Part model, mm, in its own coordinate system. Face numbers are marked on the shaded views. A direction names the side the tool comes from. Round coordinates to 2 decimals unless told otherwise and drop trailing zeros. Loops run counter-clockwise (first coordinate to the right, second up) from the corner with the lowest first, then second, coordinate; pieces in that order, holes last. Notation, with made-up numbers: M -25,-4 L 17,-4 A28 cw 17,22 Z; hole C 38,-17.75 d7. An arc over 180 degrees is marked long. Put each result on its own line as item: value. Start each with the question number.
```python
from build123d import *

# Parameters (mm, degrees)
SKETCH_1_W                  = 86
SKETCH_1_H                  = 43
EXTRUDE_1_DEPTH             = 39.5
EXTRUDE_2_DEPTH             = 5
SKETCH_3_W                  = 80.6
SKETCH_3_H                  = 40.2
CUT_EXTRUDE_1_DEPTH         = 43.6
HOLE_WIZARD_8_3_8_3_1_D     = 8.3
HOLE_WIZARD_8_3_8_3_1_DEPTH = 3.2
FILLET_1_R                  = 3
EXTRUDE_START               = -4
SKETCH_6_R                  = 4.15
EXTRUDE_3_DEPTH             = 4
SKETCH_10_W                 = 2.2
SKETCH_10_H                 = 43
EXTRUDE_5_DEPTH             = 42
FILLET_2_R                  = 2


with BuildPart() as part:
    # Эскиз1 → Бобышка-Вытянуть1 (new body)
    with BuildSketch(Plane.XY.offset(22.25)):
        with Locations((47, 0)):
            Rectangle(SKETCH_1_W, SKETCH_1_H)
    extrude(amount=-EXTRUDE_1_DEPTH)

    # Эскиз2 → Бобышка-Вытянуть2 (add)
    with BuildSketch(Plane(origin=(0, 0, -17.25), x_dir=(-1, 0, 0), z_dir=(0, 0, -1))):
        with BuildLine():
            Line((-90, -21.5), (-90, -16.5))
            ThreePointArc((-90, -16.5), (-104, 0), (-90, 16.5))
            Line((-90, 16.5), (-90, 21.5))
            Line((-90, 21.5), (-4, 21.5))
            Line((-4, 21.5), (-4, -21.5))
            Line((-4, -21.5), (-90, -21.5))
        make_face()
        with BuildLine():
            Line((-90, -12.428366172), (-90, 12.428366172))
            ThreePointArc((-90, 12.428366172), (-100, 0), (-90, -12.428366172))
        make_face(mode=Mode.SUBTRACT)
    extrude(amount=EXTRUDE_2_DEPTH)

    # Эскиз3 → Вырез-Вытянуть1 (cut)
    with BuildSketch(Plane.XY.offset(22.25)):
        with Locations((48.3, 0)):
            Rectangle(SKETCH_3_W, SKETCH_3_H)
    extrude(amount=-CUT_EXTRUDE_1_DEPTH, mode=Mode.SUBTRACT)

    # Диаметр отверстия Ø8.3 (8.3)1
    with Locations(Plane.ZY.offset(-4)):
        with Locations((0, 0)):
            Hole(HOLE_WIZARD_8_3_8_3_1_D / 2, depth=HOLE_WIZARD_8_3_8_3_1_DEPTH)

    # Скругление1
    fillet_1_edges = [part.edges().sort_by_distance(p)[0] for p in [
        (4, -21.5, 0),
        (4, 21.5, 0),
    ]]
    fillet(fillet_1_edges, radius=FILLET_1_R)

    # Эскиз6 → Бобышка-Вытянуть3 (add)
    with BuildSketch(Plane.ZY.offset(-4).offset(EXTRUDE_START)):
        Circle(SKETCH_6_R)
    extrude(amount=EXTRUDE_3_DEPTH)

    # Эскиз10 → Бобышка-Вытянуть5 (add)
    with BuildSketch(Plane(origin=(0, 0, -22.25), x_dir=(-1, 0, 0), z_dir=(0, 0, -1))):
        with Locations((-47.4, 0)):
            Rectangle(SKETCH_10_W, SKETCH_10_H)
    extrude(amount=-EXTRUDE_5_DEPTH)

    # Скругление2
    fillet_2_edges = [part.edges().sort_by_distance(p)[0] for p in [
        (27.15, -20.1, -21.35),
        (88.6, -20.1, 0.45),
        (8, 0, -21.35),
        (8, -20.1, 0.45),
        (68.55, 20.1, -21.35),
        (8, 20.1, 0.45),
        (88.6, 0, -21.35),
        (68.55, -20.1, -21.35),
        (27.15, 20.1, -21.35),
        (48.5, 0, -21.35),
        (46.3, 0, -21.35),
        (90, 21.5, 0),
        (46.3, -20.1, -0.8),
        (46.3, 20.1, -0.8),
        (48.5, -20.1, -0.8),
        (48.5, 20.1, -0.8),
    ]]
    fillet(fillet_2_edges, radius=FILLET_2_R)


solid = part.part
```
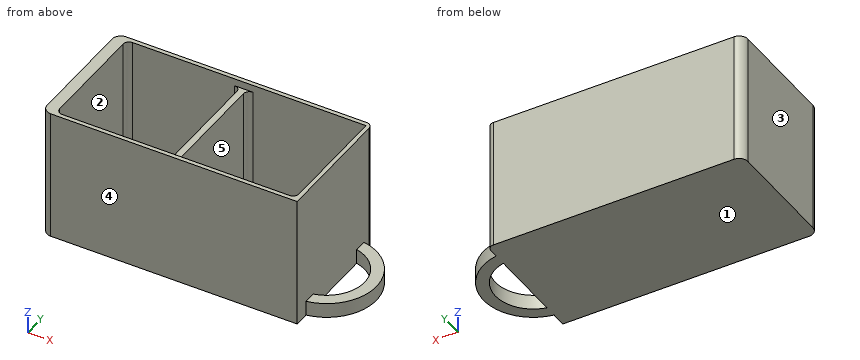
1. Cut at B-B, the plane y = 7. Give the cut face in (x, z).
2. Mould opens along X. For the marked faces 3, 4 and 5 say: released by +X, released by -X, zero draft, split by the parting line, or undercut.
3. Cut at C-C, the plane x = 72.5. Give the cut face in (y, z), and give its area (3 significant figures).
4. Cut at A-A, the plane z = -12. Give the cut face in (x, y).
5. Wall check: L1, parallel to X at y = 2.5, z = -10; L2, parallel to Y at x = 40.5, z = 8.5; L3, parallel to Z at x = 32.5, y = 12. Give the ranges that are in metal, low to high.
6. Which spindle directions (+Z, -Z, +X, -X, +Y, -Y) get a long thin tool onto all of the face, cutting with end or side? Do the marked faces 1 and 2. Say none if no direction does.
7. Drop flat-ended pins along their axis: pin 1 (18 mm diameter, centred on x = 59.5, y = 6.5, fed in from +Z); pin 2 (1 mm diameter, centred on y = 16, z = 14, fed in from +X); pin 3 (5 mm diameter, centred on x = 47, y = -1.5, fed in from +Z). Give the stop position or say it passes through.
8. Cut at D-D, the plane y = -13.5. Give the cut face in (x, z).
Results list:
1. outline: M 4,-22.25 L 90,-22.25 L 90,22.25 L 88.6,22.25 L 88.6,-19.35 A2 cw 86.6,-21.35 L 50.5,-21.35 A2 cw 48.5,-19.35 L 48.5,19.75 L 46.3,19.75 L 46.3,-19.35 A2 cw 44.3,-21.35 L 10,-21.35 A2 cw 8,-19.35 L 8,22.25 L 4,22.25 Z; M 97.9,-22.25 L 102.46,-22.25 L 102.46,-17.25 L 97.9,-17.25 Z
2. face 3: released by -X
2. face 4: zero draft
2. face 5: undercut
3. outline: M -21.5,-22.25 L 21.5,-22.25 L 21.5,22.25 L 20.1,22.25 L 20.1,-19.35 A2 cw 18.1,-21.35 L -18.1,-21.35 A2 cw -20.1,-19.35 L -20.1,22.25 L -21.5,22.25 Z
3. area: 162 mm^2
4. outline: M 4,-18.5 A3 ccw 7,-21.5 L 90,-21.5 L 90,19.5 A2 ccw 88,21.5 L 7,21.5 A3 ccw 4,18.5 Z; hole M 8,-18.1 A2 ccw 10,-20.1 L 44.3,-20.1 A2 ccw 46.3,-18.1 L 46.3,18.1 A2 ccw 44.3,20.1 L 10,20.1 A2 ccw 8,18.1 Z; hole M 48.5,-18.1 A2 ccw 50.5,-20.1 L 86.6,-20.1 A2 ccw 88.6,-18.1 L 88.6,20.1 L 50.5,20.1 A2 ccw 48.5,18.1 Z
5. L1: x = 4 to 8, 46.3 to 48.5, 88.6 to 90
5. L2: y = -21.5 to -20.1, 20.1 to 21.5
5. L3: z = -22.25 to -21.35
6. face 1: -Z, +X, -X, +Y, -Y
6. face 2: +Z
7. pin 1: stops at z = -21.35
7. pin 2: stops at x = 90
7. pin 3: stops at z = 19.75
8. outline: M 4,-22.25 L 97.15,-22.25 L 97.15,-17.25 L 90,-17.25 L 90,22.25 L 88.6,22.25 L 88.6,-19.35 A2 cw 86.6,-21.35 L 50.5,-21.35 A2 cw 48.5,-19.35 L 48.5,19.75 L 46.3,19.75 L 46.3,-19.35 A2 cw 44.3,-21.35 L 10,-21.35 A2 cw 8,-19.35 L 8,22.25 L 4,22.25 Z
